from build123d import *

# Parameters (mm, degrees)
BOSS_EXTRUDE1_DEPTH = 12.7
SKETCH2_W           = 19.05
SKETCH2_H           = 19.05
CUT_EXTRUDE1_DEPTH  = 112.125209326


with BuildPart() as part:
    # Sketch1 → Boss-Extrude1 (new, symmetric)
    with BuildSketch(Plane.XY):
        Polygon((-12.7, -54.832089482), (12.7, -45.587245531), (12.7, 54.832089482), (-12.7, 54.832089482), align=None)
    extrude(amount=BOSS_EXTRUDE1_DEPTH, both=True)

    # Sketch2 → Cut-Extrude1 (cut, through all)
    with BuildSketch(Plane(origin=(0, 54.832089482, 0), x_dir=(1, 0, 0), z_dir=(0, 1, 0))):
        Rectangle(SKETCH2_W, SKETCH2_H)
    extrude(amount=-CUT_EXTRUDE1_DEPTH, mode=Mode.SUBTRACT)


solid = part.part
Design review of the part built by this model. Coordinates are the model's own, in mm. A direction names the side the tool comes from. Give positions to 0.01 mm unless a question says otherwise; leave off trailing zeros. Write each loop counter-clockwise with the first axis right and the second up, starting at its lowest first coordinate (ties: lowest second). Pieces come first, ordered by that corner, then holes. Notation, with made-up numbers: M 21,-5.75 L 58,-5.75 A8 cw 58,-1.75 Z; hole C -23.75,78.5 d9. An arc over 180 degrees is marked long. Return JSON: item names as keys, results as strings. Group by question number.
Item 1: The part is to be moulded in two halves that separate along Z. For faces 1 (the flat face through (0, 1, 12.7)), 2 (the flat face through (-11, 54.832, 0)), 3 (the flat face through (-9.525, 1, 0)), say which applies: pulls with the +Z half, pulls with the -Z half, needs draft (parallel to the pull), parting line crosses it, or undercut.
Item 2: Take a section at B-B (z = 5). Give the boundary of the cut face in (x, y) (3 decimals).
Item 3: Take a section at A-A (y = 25.5). Give the boundary of the cut face in (x, z) (3 decimals).
Item 4: Take a section at C-C (x = -2.75). Give the boundary of the cut face in (y, z) (3 decimals), plus the area to 3 significant figures.
Item 5: Clearance check with flat-ended pins moving along their axes: pin 1 Ø1 at (x, z) = (9.5, 6.5) entering from -Y; pin 2 Ø4 at (x, z) = (-9, -3) entering from -Y. State where each tip first meets the part, or that it passes through.
Item 6: Tool access review of faces 4 (the flat face through (0, 1, 9.525)), 5 (the flat face through (12.7, 4, 0)): name each direction out of +Z, -Z, +X, -X, +Y, -Y from which nothing blocks a thin tool from reaching the whole face with its end or side.
Item 7: Take a section at D-D (z = 11). Give the boundary of the cut face in (x, y), plus the area to 3 significant figures.
Item 8: Wall thickness on line 1 along X through (y, z) = (22.5, 3.75) (3 decimals); line 2 along Y through (x, z) = (0, 11): over which ranges is each line inside the solid? List them lowest first.
Return value:
{
 "1": {"face 1": "pulls with the +Z half", "face 2": "needs draft", "face 3": "undercut"},
 "2": {"outline": "M -12.7,-54.832 L -9.525,-53.676 L -9.525,54.832 L -12.7,54.832 Z; M 9.525,-46.743 L 12.7,-45.587 L 12.7,54.832 L 9.525,54.832 Z"},
 "3": {"outline": "M -12.7,-12.7 L 12.7,-12.7 L 12.7,12.7 L -12.7,12.7 Z; hole M -9.525,-9.525 L 9.525,-9.525 L 9.525,9.525 L -9.525,9.525 Z"},
 "4": {"outline": "M -51.211,-12.7 L 54.832,-12.7 L 54.832,-9.525 L -51.211,-9.525 Z; M -51.211,9.525 L 54.832,9.525 L 54.832,12.7 L -51.211,12.7 Z", "area": "673 mm2"},
 "5": {"pin 1": "stops at y = -46.74", "pin 2": "stops at y = -54.21"},
 "6": {"face 4": "+Y, -Y", "face 5": "+Z, -Z, +X, +Y, -Y"},
 "7": {"outline": "M -12.7,-54.83 L 12.7,-45.59 L 12.7,54.83 L -12.7,54.83 Z", "area": "2,670 mm2"},
 "8": {"line 1": "x = -12.7 to -9.525, 9.525 to 12.7", "line 2": "y = -50.21 to 54.83"}
}
